Can you work these out from the drawing? Everything is in mm from the part's minimum corner. A direction names the side the tool comes from. Round coordinates to 2 decimals unless told otherwise and drop trailing zeros. Loops run counter-clockwise (first coordinate to the right, second up) from the corner with the lowest first, then second, coordinate; pieces in that order, holes last. Notation, with made-up numbers: (10.5, 6) -> (33.5, 6) arc R21 ccw to (33.5, 10) -> close; hole circle Ø4 at (79.5, 1.25). An arc over 180 degrees is marked (long way). One line per item, written item: value.
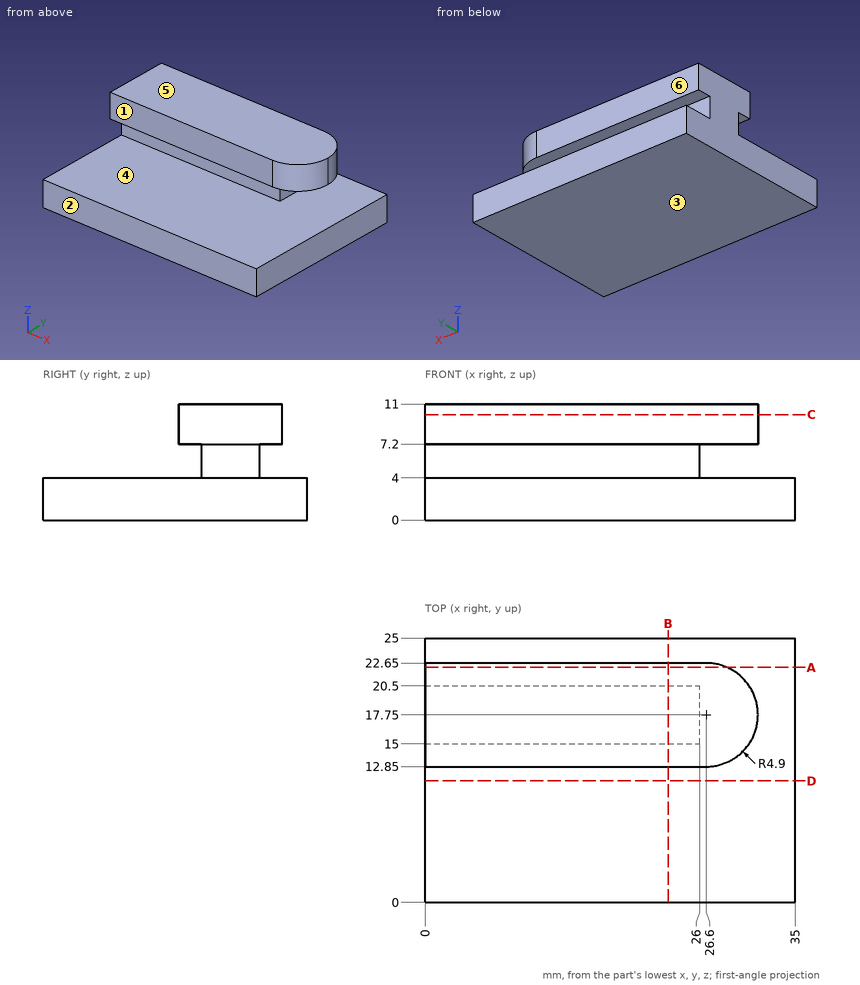
Item 1: If we section it at B-B on x = 23: List the corners of the cut face in (y, z) for me.
Output:
outline: (0, 0) -> (25, 0) -> (25, 4) -> (20.5, 4) -> (20.5, 7.2) -> (22.65, 7.2) -> (22.65, 11) -> (12.85, 11) -> (12.85, 7.2) -> (15, 7.2) -> (15, 4) -> (0, 4) -> close
Item 2: Will these pins go through, and if not, where does the flat tip stop? pin 1 Ø3.5 at (y, z) = (17, 6) entering from +X; pin 2 Ø1.5 at (x, z) = (31, 5) entering from -Y; pin 3 Ø4 at (x, y) = (30, 3) entering from +Z; pin 4 Ø6 at (y, z) = (20, 6.5) entering from -X.
Output:
pin 1: stops at x = 31.5
pin 2: passes through
pin 3: stops at z = 4
pin 4: stops at x = 0
Item 3: If we section it at D-D on y = 11.5: List the corners of the cut face in (x, z) for me, plus the area to 3 significant figures.
Output:
outline: (0, 0) -> (35, 0) -> (35, 4) -> (0, 4) -> close
area: 140 mm²
Item 4: For the marked faces 1 and 2, which set-ups out of +Z, -Z, +X, -X, +Y, -Y let a thin tool reach every point of the face, with its end or its side?
Output:
face 1: +Z, +X, -X, -Y
face 2: +Z, -Z, +X, -X, -Y
Item 5: If we mould it in two halves opening along Z, with no side actions, what happens to the marked faces 3, 4, 5 and 6? For each: released by +Z, released by -Z, zero draft, split by the parting line, or undercut.
Output:
face 3: released by -Z
face 4: undercut
face 5: released by +Z
face 6: zero draft
Item 6: If we section it at A-A on y = 22.25: List the corners of the cut face in (x, z) for me, plus the area to 3 significant figures.
Output:
outline: (0, 0) -> (35, 0) -> (35, 4) -> (0, 4) -> close; (0, 7.2) -> (28.54, 7.2) -> (28.54, 11) -> (0, 11) -> close
area: 248 mm²
Item 7: I need wall thicknesses on line 1 (Z direction, x = 30, y = 20.5); line 2 (Z direction, x = 33, y = 9.5); line 3 (Y direction, x = 23.5, z = 4.25). Which ranges of each line are inside material? Lowest first, please. Write a range as from..to.
Output:
line 1: z = 0..4, 7.2..11
line 2: z = 0..4
line 3: y = 15..20.5
Item 8: If we section it at C-C on z = 10: List the corners of the cut face in (x, y) for me, plus the area to 3 significant figures.
Output:
outline: (0, 12.85) -> (26.6, 12.85) arc R4.9 ccw to (31.5, 17.75) arc R4.9 ccw to (26.6, 22.65) -> (0, 22.65) -> close
area: 298 mm²
